```python
from build123d import *

# Parameters (mm, degrees)
SKETCH1_W           = 70
SKETCH1_H           = 100
SKETCH1_W_2         = 10
SKETCH1_H_2         = 3
BOSS_EXTRUDE1_DEPTH = 3
SKETCH2_W           = 10
SKETCH2_H           = 3
CUT_EXTRUDE1_DEPTH  = 64.584589328


with BuildPart() as part:
    # Sketch1 → Boss-Extrude1 (new body)
    with BuildSketch(Plane.XY):
        Rectangle(SKETCH1_W, SKETCH1_H)
        with Locations((21.5, -51.5)):
            Rectangle(SKETCH1_W_2, SKETCH1_H_2)
        with Locations((1.5, -51.5)):
            Rectangle(SKETCH1_W_2, SKETCH1_H_2)
        with Locations((-18.5, -51.5)):
            Rectangle(SKETCH1_W_2, SKETCH1_H_2)
    extrude(amount=BOSS_EXTRUDE1_DEPTH)

    # Sketch2 → Cut-Extrude1 (cut, through all)
    with BuildSketch(Plane.XY.offset(3)):
        with Locations((-20, 48.5)):
            Rectangle(SKETCH2_W, SKETCH2_H)
        with Locations((0, 48.5)):
            Rectangle(SKETCH2_W, SKETCH2_H)
        with Locations((20, 48.5)):
            Rectangle(SKETCH2_W, SKETCH2_H)
    extrude(amount=-CUT_EXTRUDE1_DEPTH, mode=Mode.SUBTRACT)


solid = part.part
```
Can you work these out from the model? Positions are in its coordinate system, mm. A direction names the side the tool comes from. Round coordinates to 2 decimals unless told otherwise and drop trailing zeros. Order: outer loops, then holes, each group sorted by start corner. A loop starts at its lowest first (then second) coordinate and runs counter-clockwise, first axis right, second up. Notation, with made-up numbers: (-4, 25) -> (5, 25) arc R24 ccw to (5, 59) -> close; hole circle Ø2 at (-10.5, 63.25). An arc over 180 degrees is marked (long way). Return JSON: item names as keys, results as strings. Group by question number.
1. Will these pins go through, and if not, where does the flat tip stop? pin 1 (1.5 mm diameter, centred on x = -2.5, z = 2, fed in from +Y); pin 2 (0.9 mm diameter, centred on x = -7, z = 1, fed in from -Y); pin 3 (1.5 mm diameter, centred on y = -52, z = 1.5, fed in from +X).
2. I need wall thicknesses on line 1 (Y direction, x = 3, z = 0.75); line 2 (Y direction, x = -24, z = 0.6). Which ranges of each line are inside material? Lowest first, please. Write a range as [from, to].
3. We'd pull the mould along X, two halves only. Please class faces 1 (the face through (10, 50, 1)), 2 (the face through (26.5, -52, 1)), 3 (the face through (-3.5, -52, 1)): released by +X, released by -X, zero draft, split by the parting line, or undercut.
4. Which directions (+Z, -Z, +X, -X, +Y, -Y) give clear straight access to the entire face, cutting with the end or side of a thin tool? Please do faces 4 (the face through (6.5, -52, 1)), 5 (the face through (-29, -50, 1)), 6 (the face through (31, -50, 1)), 7 (the face through (5, 48, 2)).
5. If we section it at B-B, the plane x = 9: Write out the boundary of the cut face in (y, z).
6. If we section it at A-A, the plane z = 1.75: Write out the boundary of the cut face in (x, y), then the cut area to 3 significant figures.
Output values:
{
 "1": {"pin 1": "y = 47", "pin 2": "y = -50", "pin 3": "x = 26.5"},
 "2": {"line 1": "[-53, 47]", "line 2": "[-50, 47]"},
 "3": {"face 1": "zero draft", "face 2": "released by +X", "face 3": "undercut"},
 "4": {"face 4": "+Z, -Z, -Y", "face 5": "+Z, -Z, -X, -Y", "face 6": "+Z, -Z, +X, -Y", "face 7": "+Z, -Z, +Y"},
 "5": {"outline": "(-50, 0) -> (50, 0) -> (50, 3) -> (-50, 3) -> close"},
 "6": {"outline": "(-35, -50) -> (-23.5, -50) -> (-23.5, -53) -> (-13.5, -53) -> (-13.5, -50) -> (-3.5, -50) -> (-3.5, -53) -> (6.5, -53) -> (6.5, -50) -> (16.5, -50) -> (16.5, -53) -> (26.5, -53) -> (26.5, -50) -> (35, -50) -> (35, 50) -> (25, 50) -> (25, 47) -> (15, 47) -> (15, 50) -> (5, 50) -> (5, 47) -> (-5, 47) -> (-5, 50) -> (-15, 50) -> (-15, 47) -> (-25, 47) -> (-25, 50) -> (-35, 50) -> close", "area": "7,000 mm²"}
}
